Geometry check sheet. Reference: the model listing, model coordinates, mm. A direction names the side the tool comes from. Give positions to 0.01 mm unless a question says otherwise; leave off trailing zeros. Order: outer loops, then holes, each group sorted by start corner. A loop starts at its lowest first (then second) coordinate and runs counter-clockwise, first axis right, second up. Notation, with made-up numbers: (62.5, 82.25) - (109.5, 82.25) arc R27 cw to (109.5, 100.25) - close; hole circle Ø4 at (70, 31). An arc over 180 degrees is marked (long way). Put each result on its own line as item: value. Start each with the question number.
Autodesk Inventor part; units mm, degrees
ref_plane "YZ Plane" through (0, 0, 0) normal (1, 0, 0) x (0, 1, 0)
ref_plane "XZ Plane" through (0, 0, 0) normal (0, 1, 0) x (-1, 0, 0)
ref_plane "XY Plane" through (0, 0, 0) normal (0, 0, 1) x (1, 0, 0)
sketch "Sketch1" plane through (0, 0, 0) normal (0, 1, 0) x (-1, 0, 0)
  line L0 (-80, 117) -> (80, 117)
  line L1 (80, 117) -> (80, -117)
  line L2 (80, -117) -> (-80, -117)
  line L3 (-80, -117) -> (-80, 117)
  line L4 (-80, 117) -> (80, -117) construction
  line L5 (80, 117) -> (-80, -117) construction
  point P0 (0, 0)
  dimension "d0" = 160
  dimension "d1" = 234
extrude "Extrusion1" add sketch "Sketch1" along normal blind 6
sketch "Sketch2" plane through (0, 6, 0) normal (0, 1, 0) x (1, 0, 0)
  line L0 (80, 117) -> (-80, 117)
  line L1 (-80, 117) -> (-80, -117)
  line L2 (-80, -117) -> (80, -117)
  line L3 (80, -117) -> (80, 117)
  line L4 (76.2612, -82.1) -> (62.1597, -82.1)
  line L5 (62.1597, 116.5) -> (62.1597, -117.5)
  line L6 (62.1597, -82.1) -> (70.1597, -82.1)
  line L7 (70.1597, -82.1) -> (70.1597, -55.7)
  line L8 (70.1597, -55.7) -> (62.1597, -55.7)
  line L9 (62.1597, -55.7) -> (62.1597, -82.1)
  line L10 (70.1597, -82.1) -> (62.1597, -82.1)
  line L11 (62.1597, -82.1) -> (62.1597, -81.1)
  line L12 (62.1597, -81.1) -> (70.1597, -81.1)
  line L13 (70.1597, -81.1) -> (70.1597, -82.1)
  point P0 (0, 0)
  point P1 (66.1597, -55.7)
  point P2 (66.1597, -82.1)
  point P3 (62.1597, -55.7)
  dimension "d4" = 26.4
  dimension "d5" = 8
  dimension "d8" = 1
extrude "Extrusion2" add sketch "Sketch2" along normal blind 25.4 contours L5 L8 L7 L12
sketch "Sketch3" plane through (70.1597, 6, 81.1) normal (1, 0, 0) x (0, 0, -1)
  line L0 (25.4, 0) -> (0, 0)
  line L1 (25.4, 0) -> (25.4, 25.4)
  line L2 (0, 25.4) -> (25.4, 25.4)
  line L3 (0, 0) -> (0, 25.4)
  circle A0 centre (12.7, 12.7) radius 2.75
  point P0 (81.1, -6)
  dimension "d9" = 5.5
extrude "Extrusion3" cut sketch "Sketch3" against normal blind 25.4 contours A0
fillet "Fillet1" radius 8 3 edges at (70.1597, 6, 68.4) (66.1597, 31.4, 55.7) (66.1597, 31.4, 81.1)
sketch "Sketch4" plane through (0, 6, 0) normal (0, 1, 0) x (1, 0, 0)
  line L0 (78.1597, -81.1) -> (62.1597, -81.1)
  line L1 (62.1597, -81.1) -> (62.1597, -55.7)
  line L2 (62.1597, -55.7) -> (78.1597, -55.7)
  line L3 (78.1597, -81.1) -> (78.1597, -55.7)
  line L4 (80, 117) -> (-80, 117)
  line L5 (-80, 117) -> (-80, -117)
  line L6 (-80, -117) -> (80, -117)
  line L7 (80, -117) -> (80, 117)
  line L8 (-217.2403, -92.1) -> (36.7597, -92.1)
  line L9 (-7.3833, -87.6172) -> (32.2769, -47.957)
  line L10 (-13.6234, -92.1) -> (-73.3252, -92.1)
  line L11 (-73.3252, -92.1) -> (-73.3252, -84.1)
  line L12 (-73.3252, -84.1) -> (-13.6234, -84.1)
  line L13 (-13.6234, -84.1) -> (-13.6234, -92.1)
  point P0 (0, 0)
  point P1 (-73.3252, -92.1)
  dimension "d14" = 8
extrude "Extrusion4" add sketch "Sketch4" along normal blind 25.4 contours L11 L12 L13 L8
sketch "Sketch5" plane through (-80, 6, 84.1) normal (0, 0, -1) x (-1, 0, 0)
  line L0 (-6.6748, 0) -> (-66.3766, 0)
  line L1 (-6.6748, 0) -> (-6.6748, 25.4)
  line L2 (-66.3766, 25.4) -> (-6.6748, 25.4)
  line L3 (-66.3766, 0) -> (-66.3766, 25.4)
  circle A0 centre (-56.0684, 12.7) radius 2.75
  circle A1 centre (-21.0684, 12.7) radius 2.75
  circle A2 centre (13.9316, 12.7) radius 2.75
  point P0 (-80, -6)
  dimension "d17" = 5.5
  dimension "d22" = 35
extrude "Extrusion5" cut sketch "Sketch5" against normal blind 25.4 contours A0 | A1 | A2
mirror "Mirror1" about plane through (0, 0, 0) normal (0, 0, 1) of "Extrusion2", "Extrusion3", "Fillet1", "Extrusion4", "Extrusion5"
sketch "Sketch6" plane through (0, 6, 0) normal (0, 1, 0) x (1, 0, 0)
  line L0 (-13.6234, 84.1) -> (-73.3252, 84.1)
  line L1 (-73.3252, 84.1) -> (-73.3252, 92.1)
  line L2 (-73.3252, 92.1) -> (-13.6234, 92.1)
  line L3 (-13.6234, 92.1) -> (-13.6234, 84.1)
  line L4 (78.1597, 55.7) -> (62.1597, 55.7)
  line L5 (62.1597, 55.7) -> (62.1597, 81.1)
  line L6 (62.1597, 81.1) -> (78.1597, 81.1)
  line L7 (78.1597, 55.7) -> (78.1597, 81.1)
  line L8 (-73.3252, -84.1) -> (-13.6234, -84.1)
  line L9 (-13.6234, -84.1) -> (-13.6234, -92.1)
  line L10 (-13.6234, -92.1) -> (-73.3252, -92.1)
  line L11 (-73.3252, -92.1) -> (-73.3252, -84.1)
  line L12 (78.1597, -81.1) -> (62.1597, -81.1)
  line L13 (62.1597, -81.1) -> (62.1597, -55.7)
  line L14 (62.1597, -55.7) -> (78.1597, -55.7)
  line L15 (78.1597, -81.1) -> (78.1597, -55.7)
  line L16 (80, 117) -> (-80, 117)
  line L17 (-80, 117) -> (-80, -117)
  line L18 (-80, -117) -> (80, -117)
  line L19 (80, -117) -> (80, 117)
  line L20 (-14.0403, 77.5) -> (-69.0403, 77.5)
  line L21 (-69.0403, 77.5) -> (-69.0403, -77.5)
  line L22 (-69.0403, -77.5) -> (-14.0403, -77.5)
  line L23 (-14.0403, -77.5) -> (-14.0403, 77.5)
  line L24 (-14.0403, 77.5) -> (-69.0403, -77.5) construction
  line L25 (-69.0403, 77.5) -> (-14.0403, -77.5) construction
  line L26 (80, -117) -> (80, 117)
  line L27 (80, 0) -> (-80, 0)
  line L28 (-9.0403, -82.5) -> (-74.0403, -82.5)
  line L29 (-74.0403, -82.5) -> (-74.0403, 82.5)
  line L30 (-74.0403, 82.5) -> (-9.0403, 82.5)
  line L31 (-9.0403, 82.5) -> (-9.0403, -82.5)
  point P0 (0, 0)
  point P1 (-41.5403, 0)
  dimension "d27" = 155
  dimension "d28" = 55
  dimension "d29" = 76.2
  dimension "d30" = 5
sketch "Sketch7" plane through (0, 6, 0) normal (0, 1, 0) x (1, 0, 0)
  line L0 (-14.0403, 77.5) -> (-69.0403, 77.5)
  line L1 (-69.0403, 77.5) -> (-69.0403, -77.5)
  line L2 (-69.0403, -77.5) -> (-14.0403, -77.5)
  line L3 (-14.0403, -77.5) -> (-14.0403, 77.5)
  point P0 (0, 0)
properties part number "lowerSkidPlate"
Item 1: Release check for a two-part mould opening along Z. For faces 1 (the face through (66.216, 28.994, -78.819)), 2 (the face through (-44, 19, 84.1)), 3 (the face through (1, 3, 117)) record: +Z half, -Z half, draft (parallel to the pull), parting line (faces both ways), or undercut.
Item 2: Cross-section at A-A (z = 68.4). Enter the section's corners in (x, y).
Item 3: Cross-section at B-B (y = 18.7). Count the separate pieces of the cut face and the enclosed holes in it, and give its area (3 significant figures).
Item 4: Cross-section at C-C (x = -5). Enter the section's corners in (y, z), and give its area (3 significant figures).
Item 5: Set-up check for faces 4 (the face through (66, 15, 81.1)), 5 (the face through (62.16, 15.7, -68.6)), 6 (the face through (70.16, 23, -68)), 7 (the face through (66.104, 29.119, 58.106)), 8 (the face through (67, 15, -81.1)): record each of +Z, -Z, +X, -X, +Y, -Y from which the full face is reachable in a straight line by a thin tool's end or side.
Item 6: Cross-section at D-D (z = -17). Enter the section's corners in (x, y), and give its area (3 significant figures).
Item 7: Thickness scan on line 1 along X through (y, z) = (18.7, -87.75); line 2 along Y through (x, z) = (65, 68); line 3 along X through (y, z) = (18, -90). Record the ranges inside material, lowest first.
Item 8: Gauge pin test, flat ends, axial feed: pin 1 Ø8 at (x, y) = (73, 18.5) entering from +Z; pin 2 Ø9 at (y, z) = (20, -88.5) entering from -X; pin 3 Ø7.5 at (x, y) = (-48, 17) entering from +Z. Record the tip position at first contact, or that the pin passes through.
Recorded:
1. face 1: -Z half
1. face 2: undercut
1. face 3: +Z half
2. outline: (-80, 0) - (80, 0) - (80, 6) - (78.16, 6) arc R8 cw to (70.16, 14) - (70.16, 15.95) - (62.16, 15.95) - (62.16, 6) - (-80, 6) - close; (62.16, 21.45) - (70.16, 21.45) - (70.16, 31.4) - (62.16, 31.4) - close
3. separate pieces: 10
3. enclosed holes: 0
3. area: 1,100 mm^2
4. outline: (0, -117) - (6, -117) - (6, 117) - (0, 117) - close
4. area: 1,400 mm^2
5. face 4: +Z, +X, -X, +Y
5. face 5: +Z, -Z, -X, +Y
5. face 6: +Z, -Z, +X, +Y
5. face 7: +X, -X, +Y
5. face 8: -Z, +X, -X, +Y
6. outline: (-80, 0) - (80, 0) - (80, 6) - (-80, 6) - close
6. area: 960 mm^2
7. line 1: x = -73.33 to -61.68, -56.18 to -26.68, -21.18 to -13.62
7. line 2: y = 0 to 15.98, 21.42 to 31.4
7. line 3: x = -73.33 to -61.59, -56.27 to -26.59, -21.27 to -13.62
8. pin 1: stops at z = 81.1
8. pin 2: stops at x = -73.33
8. pin 3: stops at z = 92.1
